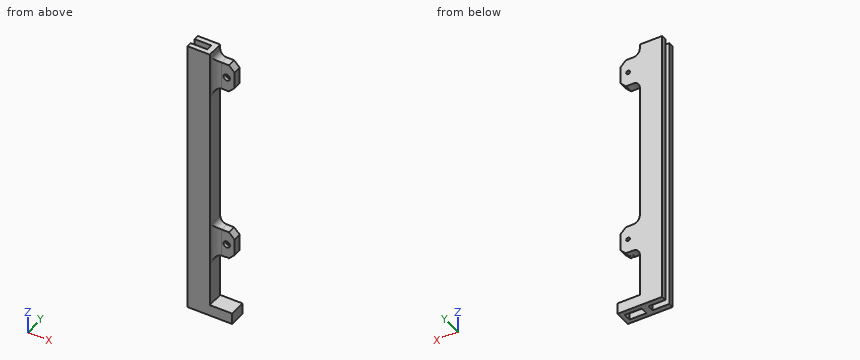
Autodesk Inventor part; units mm, degrees
ref_plane "Work Plane1" through (0, 0, 330) normal (0, 0, 1) x (1, 0, 0)
ref_plane "YZ Plane" through (0, 0, 0) normal (1, 0, 0) x (0, 1, 0)
ref_plane "XZ Plane" through (0, 0, 0) normal (0, 1, 0) x (-1, 0, 0)
sketch "Sketch1" plane through (0, 0, 0) normal (0, 0, 1) x (1, 0, 0)
  line L0 (-7.5, 2.9) -> (7.5, 2.9)
  line L1 (7.5, 2.9) -> (7.5, -2.9)
  line L2 (7.5, -2.9) -> (-7.5, -2.9)
  line L3 (-7.5, -2.9) -> (-7.5, 2.9)
  line L4 (-7.5, 2.9) -> (7.5, -2.9) construction
  line L5 (7.5, 2.9) -> (-7.5, -2.9) construction
  line L6 (-12.5, 7.5) -> (12.5, 7.5)
  line L7 (12.5, 7.5) -> (12.5, -7.5)
  line L8 (12.5, -7.5) -> (-12.5, -7.5)
  line L9 (-12.5, -7.5) -> (-12.5, 7.5)
  line L10 (-12.5, 7.5) -> (12.5, -7.5) construction
  line L11 (12.5, 7.5) -> (-12.5, -7.5) construction
  line L12 (-7.5, 7.5) -> (-7.5, -7.5)
  point P0 (0, 0)
  point P1 (-7.5, 2.9)
  dimension "d0" = 15
  dimension "d1" = 5.8
  dimension "d2" = 25
  dimension "d3" = 15
extrude "Extrusion1" add sketch "Sketch1" along normal blind 500 contours L12 L6 L7 L8 L2 L1 L0
ref_plane "Work Plane1" through (0, 0, 330) normal (0, 0, 1) x (1, 0, 0)
sketch "Sketch2" plane through (0, 0, 330) normal (0, 0, 1) x (1, 0, 0)
  line L0 (-5, 7.5) -> (30, 7.5)
  line L1 (30, 7.5) -> (30, -7.5)
  line L2 (30, -7.5) -> (-5, -7.5)
  line L3 (-5, -7.5) -> (-5, 7.5)
  line L4 (12.5, -7.5) -> (12.5, 7.5)
  line L5 (-5, 7.5) -> (30, -7.5) construction
  line L6 (30, 7.5) -> (-5, -7.5) construction
  line L7 (12.5, 0) -> (30, 0)
  line L8 (30, 0) -> (30, 7.5)
  line L9 (30, 7.5) -> (12.5, 7.5)
  line L10 (12.5, 7.5) -> (12.5, 0)
  line L11 (7.5, -2.9) -> (-7.5, -2.9)
  line L12 (-7.5, -2.9) -> (-7.5, -7.5)
  line L13 (-7.5, -7.5) -> (12.5, -7.5)
  line L14 (12.5, -7.5) -> (12.5, 7.5)
  line L15 (12.5, 7.5) -> (-7.5, 7.5)
  line L16 (-7.5, 7.5) -> (-7.5, 2.9)
  line L17 (-7.5, 2.9) -> (7.5, 2.9)
  line L18 (7.5, 2.9) -> (7.5, -2.9)
  point P0 (0, 0)
  point P1 (12.5, -6.5)
  point P2 (12.5, 6.5)
  point P3 (12.5, 7.5)
  point P4 (12.5, 6.5)
  point P5 (30, 0)
  dimension "d8" = 35
extrude "Extrusion2" add sketch "Sketch2" against normal blind 25 contours L0 L1 L7 L4
fillet "Fillet2" radius 6 3 edges at (12.5, 3.75, 305) (12.5, 0, 317.5) (12.5, 3.75, 330)
sketch "Sketch4" plane through (-7.5, 7.5, 0) normal (0, 1, 0) x (1, 0, 0)
  line L0 (20, 0) -> (0, 0)
  line L1 (0, 0) -> (0, -500)
  line L2 (20, -500) -> (0, -500)
  line L3 (20, -336) -> (20, -500)
  arc A0 (26, -330) -> (20, -336) centre (26, -336) ccw
  line L4 (37.5, -330) -> (26, -330)
  line L5 (37.5, -330) -> (37.5, -305)
  line L6 (26, -305) -> (37.5, -305)
  arc A1 (20, -299) -> (26, -305) centre (26, -299) ccw
  line L7 (20, 0) -> (20, -299)
  circle A2 centre (30.5, -317.5) radius 1.65
  line L8 (20, 0) -> (20, -500)
  line L9 (20, -250) -> (51.65, -250)
  circle A3 centre (30.5, -142.5) radius 1.65
  point P0 (7.5, 0)
  point P1 (20, -181)
  point P2 (20, -144)
  point P3 (37.5, -317.5)
  point P4 (37.5, -142.5)
  dimension "d16" = 3.3
  dimension "d17" = 7
extrude "Extrusion4" cut sketch "Sketch4" against normal through all contours A2 | A3
chamfer "Chamfer1" distance 5 angle 45 2 edges at (30, 3.75, 330) (30, 3.75, 305)
sketch "Sketch5" plane through (18.5, 0, 305) normal (0, -1, 0) x (1, 0, 0)
  line L0 (11.5, -170) -> (6.5, -175)
  line L1 (11.5, -170) -> (11.5, -155)
  line L2 (6.5, -150) -> (11.5, -155)
  line L3 (0, -150) -> (6.5, -150)
  line L4 (0, -175) -> (0, -150)
  line L5 (6.5, -175) -> (0, -175)
  circle A0 centre (4.5, -162.5) radius 1.65
  circle A1 centre (4.5, 12.5) radius 1.65
  line L6 (11.5, 5) -> (6.5, 0)
  line L7 (11.5, 20) -> (11.5, 5)
  line L8 (6.5, 25) -> (11.5, 20)
  line L9 (0, 25) -> (6.5, 25)
  line L10 (0, 0) -> (0, 25)
  line L11 (6.5, 0) -> (0, 0)
  circle A2 centre (4.5, 12.5) radius 2.9
  circle A3 centre (4.5, -162.5) radius 2.9
  point P0 (-18.5, -305)
  dimension "d23" = 5.8
extrude "Extrusion5" cut sketch "Sketch5" against normal blind 3 contours A2 | A3
ref_plane "Work Plane3" through (0, 0, 250) normal (0, 0, -1) x (-1, 0, 0)
pattern_linear "Rectangular Pattern1" count 2 spacing 160 along (0, 0, 1) of "Extrusion2", "Fillet2", "Extrusion4", "Chamfer1", "Extrusion5"
mirror "Mirror1" about plane through (0, 0, 250) normal (0, 0, -1) of "Extrusion2", "Fillet2", "Extrusion4", "Chamfer1", "Extrusion5", "Rectangular Pattern1"
ref_plane "Work Plane4" through (0, 0, 250) normal (0, 0, 1) x (1, 0, 0)
sketch "Sketch6" plane through (0, 0, 250) normal (0, 0, 1) x (1, 0, 0)
  line L0 (12.5, 7.5) -> (12.5, -6)
  line L1 (12.5, -6) -> (12.5, 7.5)
  line L2 (12.5, 7.5) -> (12.5, -6)
  line L3 (12.5, -6) -> (12.5, 7.5)
  line L4 (12.5, 7.5) -> (12.5, -6)
  line L5 (12.5, -6) -> (12.5, 7.5)
  line L6 (12.5, 7.5) -> (12.5, -6)
  line L7 (12.5, -7.5) -> (12.5, 7.5)
  line L8 (12.5, -7.5) -> (12.5, 7.5)
  line L9 (12.5, -6) -> (12.5, 7.5)
  line L10 (12.5, 7.5) -> (32.5, 7.5)
  line L11 (32.5, 7.5) -> (32.5, -7.5)
  line L12 (32.5, -7.5) -> (12.5, -7.5)
  line L13 (12.5, -7.5) -> (12.5, 7.5)
  point P0 (0, 0)
  dimension "d29" = 20
extrude "Extrusion6" add sketch "Sketch6" along normal mid plane 20
sketch "Sketch7" plane through (0, 0, 250) normal (0, 0, 1) x (1, 0, 0)
  line L0 (-73.1551, 38.5197) -> (60.6388, 38.5197)
  line L1 (60.6388, 38.5197) -> (60.6388, -29.4562)
  line L2 (60.6388, -29.4562) -> (-73.1551, -29.4562)
  line L3 (-73.1551, -29.4562) -> (-73.1551, 38.5197)
  point P0 (0, 0)
extrude "Extrusion7" cut sketch "Sketch7" against normal through all
sketch "Sketch8" plane through (0, 0, 250) normal (0, 0, -1) x (-1, 0, 0)
  line L0 (-7.5, 2.9) -> (-7.5, -2.9)
  line L1 (7.5, 2.9) -> (-7.5, 2.9)
  line L2 (7.5, 7.5) -> (7.5, 2.9)
  line L3 (-32.5, 7.5) -> (7.5, 7.5)
  line L4 (-32.5, -7.5) -> (-32.5, 7.5)
  line L5 (7.5, -7.5) -> (-32.5, -7.5)
  line L6 (7.5, -2.9) -> (7.5, -7.5)
  line L7 (-7.5, -2.9) -> (7.5, -2.9)
  line L8 (-28.5, 3.5) -> (-13.5, 3.5)
  line L9 (-13.5, 3.5) -> (-13.5, -3.5)
  line L10 (-13.5, -3.5) -> (-28.5, -3.5)
  line L11 (-28.5, -3.5) -> (-28.5, 3.5)
  point P0 (0, 0)
  point P1 (-28.5, 0)
  point P2 (-32.5, 0)
  dimension "d34" = 4
  dimension "d35" = 15
  dimension "d36" = 7
extrude "Extrusion8" cut sketch "Sketch8" against normal blind 6 contours L8 L9 L10 L11
properties part number "GUIA DE TAPA PRINCIPAL"
Design review of the part built by this model. Coordinates are the model's own, in mm. Give positions to 0.01 mm unless a question says otherwise; leave off trailing zeros. Order: outer loops, then holes, each group sorted by start corner. A loop starts at its lowest first (then second) coordinate and runs counter-clockwise, first axis right, second up. Notation, with made-up numbers: (22.5, -21) -> (60.5, -21) arc R35 cw to (60.5, 16) -> close; hole circle Ø3 at (-10, 4.25). An arc over 180 degrees is marked (long way). Write item = value, one per line. Start each with the question number.
(1) For pin 1 (9 mm diameter, centred on x = 27, z = 323.5, fed in from -Y); pin 2 (5 mm diameter, centred on x = 20, y = 3.5, fed in from +Z); pin 3 (2 mm diameter, centred on y = 3, z = 315, fed in from +X), all flat-tipped, find the tip position at first contact; note any pin that passes through.
(2) We need section A-A on z = 359. Write out the cut boundary in (x, y).
(3) To check wall thickness, follow line 1 along Z through (x, y) = (23, 1.35); line 2 along Z through (x, y) = (23, 5.1); line 3 along X through (y, z) = (2.05, 477.5). State the ranges of each line that lie inside material, in increasing order.
Numbers:
q1.pin_1 = 0
q1.pin_2 = 490.08
q1.pin_3 = 30
q2.outline = (-7.5, -7.5) -> (12.5, -7.5) -> (12.5, 7.5) -> (-7.5, 7.5) -> (-7.5, 2.9) -> (7.5, 2.9) -> (7.5, -2.9) -> (-7.5, -2.9) -> close
q3.line_1 = 256 to 260, 305.4 to 314.6, 320.4 to 330, 465 to 474.6, 480.4 to 490
q3.line_2 = 250 to 260, 305 to 315.85, 319.15 to 330, 465 to 475.85, 479.15 to 490
q3.line_3 = 7.5 to 20.1, 25.9 to 30
